Source: three-view drawing plus pictorial views. Frame: mm from the lowest corner of the part. A direction names the side the tool comes from. Coordinates: 2 decimals unless noted, no trailing zeros. Write each loop counter-clockwise with the first axis right and the second up, starting at its lowest first coordinate (ties: lowest second). Pieces come first, ordered by that corner, then holes. Notation, with made-up numbers: (48.5, 70.25) - (75.5, 70.25) arc R22 ccw to (75.5, 106.25) - close; hole circle Ø3 at (89.25, -17.5). An arc over 180 degrees is marked (long way). Put each result on its own line as item: value.
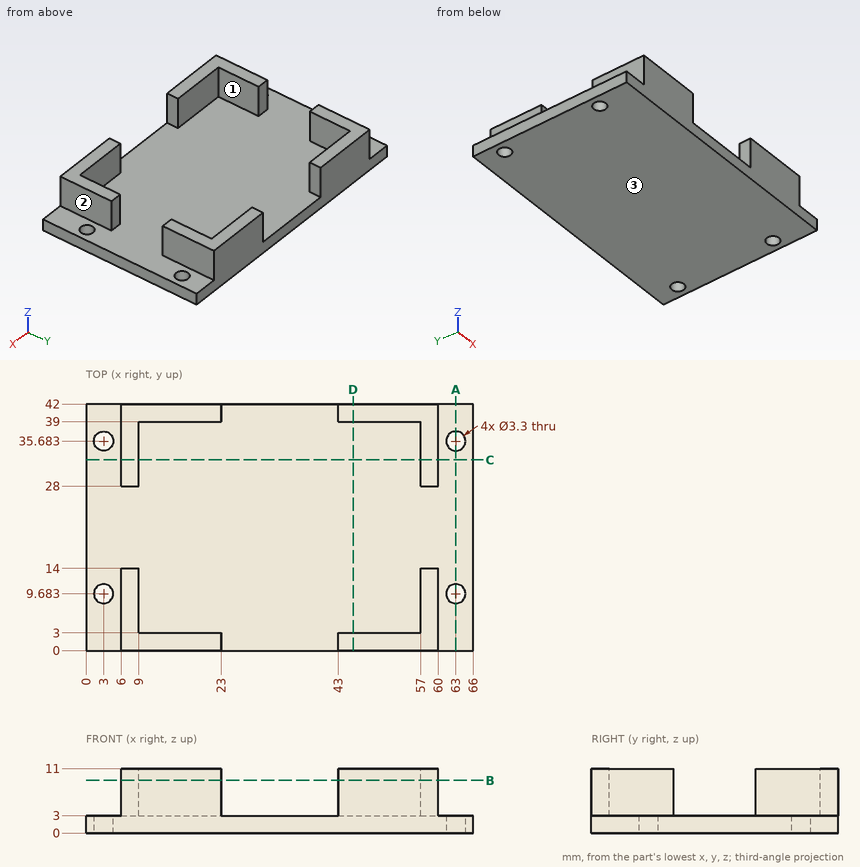
1. Section query D-D (x = 45.5). Return loops of the section in (y, z), then the cut area to 3 significant figures.
Answer below:
outline: (0, 0) - (42, 0) - (42, 11) - (39, 11) - (39, 3) - (3, 3) - (3, 11) - (0, 11) - close
area: 174 mm²
2. Ray query, probe 1 along Y at (x, z) = (63, 1.1); probe 2 along Y at (x, z) = (20.5, 5.75); probe 3 along X at (y, z) = (37, 4.5). Return the intervals inside material, ascending. Write a range as from..to.
Answer below:
probe 1: y = 0..8.03, 11.33..34.03, 37.33..42
probe 2: y = 0..3, 39..42
probe 3: x = 6..9, 57..60
3. Pin query (flat end, axial travel): pin 1 Ø3 at (x, y) = (19.5, 17.5) entering from +Z; pin 2 Ø4 at (y, z) = (6, 8) entering from +X; pin 3 Ø1.5 at (y, z) = (2, 5) entering from -X. Return the tip coordinate at first contact, or that it passes through.
Answer below:
pin 1: stops at z = 3
pin 2: stops at x = 60
pin 3: stops at x = 6
4. Section query A-A (x = 63). Return loops of the section in (y, z).
Answer below:
outline: (0, 0) - (8.03, 0) - (8.03, 3) - (0, 3) - close; (11.33, 0) - (34.03, 0) - (34.03, 3) - (11.33, 3) - close; (37.33, 0) - (42, 0) - (42, 3) - (37.33, 3) - close
5. Section query C-C (y = 32.5). Return loops of the section in (x, z), then the cut area to 3 significant figures.
Answer below:
outline: (0, 0) - (66, 0) - (66, 3) - (60, 3) - (60, 11) - (57, 11) - (57, 3) - (9, 3) - (9, 11) - (6, 11) - (6, 3) - (0, 3) - close
area: 246 mm²
6. Set-up query: the marked faces 1, 2 and 3. Return all of +Z, -Z, +X, -X, +Y, -Y with unobstructed straight access to the full face (end or side cutting, diameter ignored); none if empty.
Answer below:
face 1: +Z
face 2: +Z, +X, +Y, -Y
face 3: -Z, +X, -X, +Y, -Y
7. Section query B-B (z = 9). Return loops of the section in (x, y), then the cut area to 3 significant figures.
Answer below:
outline: (6, 0) - (23, 0) - (23, 3) - (9, 3) - (9, 14) - (6, 14) - close; (6, 28) - (9, 28) - (9, 39) - (23, 39) - (23, 42) - (6, 42) - close; (43, 0) - (60, 0) - (60, 14) - (57, 14) - (57, 3) - (43, 3) - close; (43, 39) - (57, 39) - (57, 28) - (60, 28) - (60, 42) - (43, 42) - close
area: 336 mm²
